```python
from build123d import *

# Parameters (mm, degrees)
EXTRUDE_1_DEPTH     = 1
CUT_EXTRUDE_1_REACH = 3
SKETCH_2_R          = 1.6
CUT_EXTRUDE_2_REACH = 3
SKETCH_3_R          = 1.6
CUT_EXTRUDE_3_REACH = 3
SKETCH_4_R          = 1.6


with BuildPart() as part:
    # ｽｹｯﾁ1 → ﾎﾞｽ - 押し出し1 (new body)
    with BuildSketch(Plane(origin=(0, 0, 0), x_dir=(1, 0, 0), z_dir=(0, 1, 0))):
        Polygon((-80, -21.435935394), (-58.564064606, -58.564064606), (-21.435935394, -80), (21.435935394, -80), (58.564064606, -58.564064606), (80, -21.435935394), (80, 21.435935394), (58.564064606, 58.564064606), (21.435935394, 80), (-21.435935394, 80), (-58.564064606, 58.564064606), (-80, 21.435935394), align=None)
    extrude(amount=EXTRUDE_1_DEPTH)

    # ｽｹｯﾁ2 → ｶｯﾄ - 押し出し1 (cut, up to next)
    with BuildSketch(Plane(origin=(0, 1, 0), x_dir=(1, 0, 0), z_dir=(0, 1, 0)), mode=Mode.PRIVATE) as cut_extrude_1_sk1:
        with Locations((-35, 60.621778265)):
            Circle(SKETCH_2_R)
    cut_extrude_1_tool1 = extrude(cut_extrude_1_sk1.sketch, amount=-CUT_EXTRUDE_1_REACH, mode=Mode.PRIVATE) & part.part
    add(cut_extrude_1_tool1.solids().sort_by_distance((-35, 1, -60.621778))[0], mode=Mode.SUBTRACT)

    # ｽｹｯﾁ3 → ｶｯﾄ - 押し出し2 (cut, up to next)
    with BuildSketch(Plane(origin=(0, 1, 0), x_dir=(1, 0, 0), z_dir=(0, 1, 0)), mode=Mode.PRIVATE) as cut_extrude_2_sk1:
        with Locations((-35, -60.621778265)):
            Circle(SKETCH_3_R)
    cut_extrude_2_tool1 = extrude(cut_extrude_2_sk1.sketch, amount=-CUT_EXTRUDE_2_REACH, mode=Mode.PRIVATE) & part.part
    add(cut_extrude_2_tool1.solids().sort_by_distance((-35, 1, 60.621778))[0], mode=Mode.SUBTRACT)

    # ｽｹｯﾁ4 → ｶｯﾄ - 押し出し3 (cut, up to next)
    with BuildSketch(Plane(origin=(0, 1, 0), x_dir=(1, 0, 0), z_dir=(0, 1, 0)), mode=Mode.PRIVATE) as cut_extrude_3_sk1:
        with Locations((70, 0)):
            Circle(SKETCH_4_R)
    cut_extrude_3_tool1 = extrude(cut_extrude_3_sk1.sketch, amount=-CUT_EXTRUDE_3_REACH, mode=Mode.PRIVATE) & part.part
    add(cut_extrude_3_tool1.solids().sort_by_distance((70, 1, 0))[0], mode=Mode.SUBTRACT)


solid = part.part
```
Work out the finished part from the listing and answer in its coordinate system (mm). Coordinates: 2 decimals unless noted, no trailing zeros. Loops run counter-clockwise (first coordinate to the right, second up) from the corner with the lowest first, then second, coordinate; pieces in that order, holes last. Notation, with made-up numbers: (-14.75, 76.5) -> (33.25, 76.5) arc R10 cw to (33.25, 80.5) -> close; hole circle Ø10 at (8.5, 65.25). An arc over 180 degrees is marked (long way). Answer as CSV lines item,"result".
Q1. The part is cut by section A-A on y = 0.35. Write down the section's boundary in (x, z).
Findings:
outline,"(-80, -21.44) -> (-58.56, -58.56) -> (-21.44, -80) -> (21.44, -80) -> (58.56, -58.56) -> (80, -21.44) -> (80, 21.44) -> (58.56, 58.56) -> (21.44, 80) -> (-21.44, 80) -> (-58.56, 58.56) -> (-80, 21.44) -> close; hole circle Ø3.2 at (-35, -60.62); hole circle Ø3.2 at (-35, 60.62); hole circle Ø3.2 at (70, 0)"
Q2. The part is cut by section B-B on z = -66. Write down the section's boundary in (x, y).
Findings:
outline,"(-45.68, 0) -> (45.68, 0) -> (45.68, 1) -> (-45.68, 1) -> close"
Q3. This flat-tipped pin is pushed along its axis until it touches: pin 1 (6 mm diameter, centred on x = 55, z = -19, fed in from -Y). Where does it stop, or does it pass through?
Findings:
pin 1,"stops at y = 0"
Q4. The part is cut by section C-C on z = 50. Write down the section's boundary in (x, y).
Findings:
outline,"(-63.51, 0) -> (63.51, 0) -> (63.51, 1) -> (-63.51, 1) -> close"
Q5. Find the intervals of material crossed by probe 1 along X at (y, z) = (0.8, 0); probe 2 along Z at (x, y) = (-35, 0.6); probe 3 along Z at (x, y) = (-47, 0.45), in increasing order.
Findings:
probe 1,"x = -80 to 68.4, 71.6 to 80"
probe 2,"z = -72.17 to -62.22, -59.02 to 59.02, 62.22 to 72.17"
probe 3,"z = -65.24 to 65.24"
